Input: part model. Units: mm. Frame: model coordinates. Round coordinates to 2 decimals unless told otherwise and drop trailing zeros. Loops run counter-clockwise (first coordinate to the right, second up) from the corner with the lowest first, then second, coordinate; pieces in that order, holes last. Notation, with made-up numbers: (1.5, 75) - (21.5, 75) arc R31 ccw to (21.5, 99) - close; hole circle Ø8 at (5, 73.5). An arc over 180 degrees is marked (long way). One line per question, with ' | ' between items. Start each with the question number.
Item 1: Material intervals for line 1 along Z through (x, y) = (-19, -5); line 2 along Y through (x, z) = (-20.5, 1.75); line 3 along X through (y, z) = (10.5, 1.5), sorted ascending.
Item 2: Section B-B, the plane x = 7. Return loops of the section in (y, z), plus the area to 3 significant figures.
Item 3: Section C-C, the plane y = 9. Return loops of the section in (x, z).
Item 4: Section A-A, the plane z = 1.3. Return loops of the section in (x, y).
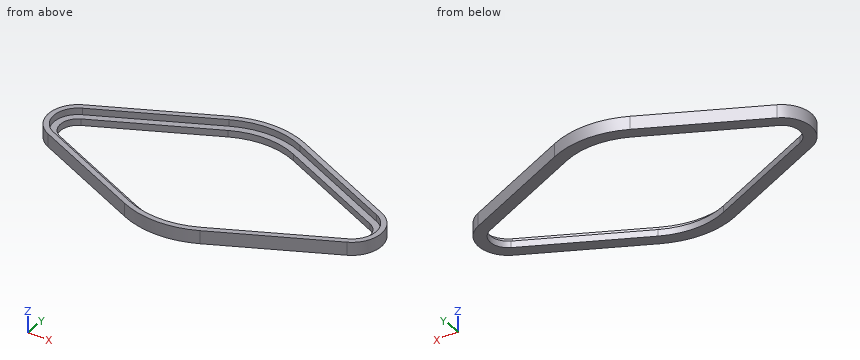
```python
from build123d import *

# Parameters (mm, degrees)
PAD_DEPTH       = 2
POCKET_DEPTH    = 1
POCKET001_DEPTH = 1.001


with BuildPart() as part:
    # Sketch → Pad (new body)
    with BuildSketch(Plane.XY):
        with BuildLine():
            Line((-22.928591, 4.065776), (-5.785719, 12.197355))
            ThreePointArc((5.785719, 12.197355), (0, 13.5), (-5.785719, 12.197355))
            Line((5.785719, 12.197355), (22.928591, 4.065776))
            ThreePointArc((22.928592, -4.065776), (25.5, 0), (22.928591, 4.065776))
            Line((22.928592, -4.065776), (5.785719, -12.197354))
            ThreePointArc((-5.785719, -12.197354), (0, -13.5), (5.785719, -12.197354))
            Line((-5.785719, -12.197354), (-22.928592, -4.065776))
            ThreePointArc((-22.928591, 4.065776), (-25.5, 0), (-22.928592, -4.065776))
        make_face()
    extrude(amount=PAD_DEPTH)

    # Sketch001 → Pocket (cut)
    with BuildSketch(Plane.XY.offset(2)):
        with BuildLine():
            Line((-22.58573, 3.342972), (-5.442864, 11.474547))
            ThreePointArc((5.442864, 11.474547), (0, 12.7), (-5.442864, 11.474547))
            Line((5.442864, 11.474547), (22.58573, 3.342972))
            ThreePointArc((22.58573, -3.342972), (24.7, 0), (22.58573, 3.342972))
            Line((22.58573, -3.342972), (5.442864, -11.474547))
            ThreePointArc((-5.442864, -11.474547), (0, -12.7), (5.442864, -11.474547))
            Line((-5.442864, -11.474547), (-22.58573, -3.342972))
            ThreePointArc((-22.58573, 3.342972), (-24.7, 0), (-22.58573, -3.342972))
        make_face()
    extrude(amount=-POCKET_DEPTH, mode=Mode.SUBTRACT)

    # Sketch002 → Pocket001 (cut, through all)
    with BuildSketch(Plane.XY.offset(1)):
        with BuildLine():
            Line((-22.157141, 2.439472), (-5.014263, 10.571053))
            ThreePointArc((5.014263, 10.571053), (0, 11.7), (-5.014263, 10.571053))
            Line((5.014263, 10.571053), (22.157141, 2.439472))
            ThreePointArc((22.157142, -2.439472), (23.7, 1e-06), (22.157141, 2.439472))
            Line((22.157142, -2.439472), (5.014261, -10.571054))
            ThreePointArc((-5.014261, -10.571054), (0, -11.7), (5.014261, -10.571054))
            Line((-5.014261, -10.571054), (-22.157142, -2.439472))
            ThreePointArc((-22.157141, 2.439472), (-23.7, 1e-06), (-22.157142, -2.439472))
        make_face()
    extrude(amount=-POCKET001_DEPTH, mode=Mode.SUBTRACT)


solid = part.part
```
Return value:
1) line 1: 0 to 1 | line 2: -5.22 to -4.33, 4.33 to 5.22 | line 3: -9.36 to -7.5, 7.5 to 9.36
2) outline: (-11.62, 0) - (-9.63, 0) - (-9.63, 1) - (-10.74, 1) - (-10.74, 2) - (-11.62, 2) - close; (9.63, 0) - (11.62, 0) - (11.62, 2) - (10.74, 2) - (10.74, 1) - (9.63, 1) - close | area: 5.76 mm2
3) outline: (-12.53, 0) - (-8.33, 0) - (-8.33, 1) - (-10.66, 1) - (-10.66, 2) - (-12.53, 2) - close; (8.33, 0) - (12.53, 0) - (12.53, 2) - (10.66, 2) - (10.66, 1) - (8.33, 1) - close
4) outline: (-22.93, -4.07) - (-5.79, -12.2) arc R13.5 ccw to (5.79, -12.2) - (22.93, -4.07) arc R4.5 ccw to (22.93, 4.07) - (5.79, 12.2) arc R13.5 ccw to (-5.79, 12.2) - (-22.93, 4.07) arc R4.5 ccw to start; hole (-22.59, -3.34) - (-5.44, -11.47) arc R12.7 ccw to (5.44, -11.47) - (22.59, -3.34) arc R3.7 ccw to (22.59, 3.34) - (5.44, 11.47) arc R12.7 ccw to (-5.44, 11.47) - (-22.59, 3.34) arc R3.7 ccw to start
